Autodesk Inventor part; units mm, degrees
ref_plane "YZ Plane" through (0, 0, 0) normal (1, 0, 0) x (0, 1, 0)
ref_plane "XZ Plane" through (0, 0, 0) normal (0, 1, 0) x (-1, 0, 0)
ref_plane "XY Plane" through (0, 0, 0) normal (0, 0, 1) x (1, 0, 0)
sketch "Sketch1" plane through (0, 0, 0) normal (0, 1, 0) x (-1, 0, 0)
  circle A0 centre (5.2854, 6.2781) radius 7.75
  point P0 (0, 0)
  dimension "d0" = 15.5
extrude "Extrusion1" add sketch "Sketch1" along normal blind 101.6
sketch "Sketch2" plane through (-5.2854, 101.6, 6.2781) normal (0, 1, 0) x (1, 0, 0)
  circle A0 centre (0, 0) radius 7.75 construction
  circle A1 centre (0, 0) radius 7
  point P0 (5.2854, 6.2781)
  dimension "d3" = 14
  dimension "d4" = 0
extrude "Extrusion2" cut sketch "Sketch2" against normal blind 101.6
sketch "Sketch3" plane through (-5.2854, 0, 6.2781) normal (0, -1, 0) x (1, 0, 0)
  circle A0 centre (0, 0) radius 7 construction
  line L0 (10, 17.5) -> (-10, 17.5)
  line L1 (-10, 17.5) -> (-10, -17.5)
  line L2 (-10, -17.5) -> (10, -17.5)
  line L3 (10, -17.5) -> (10, 17.5)
  circle A1 centre (2.5, 12) radius 2
  circle A2 centre (2.5, -12) radius 2
  point P0 (5.2854, -6.2781)
  dimension "d7" = 35
  dimension "d8" = 20
  dimension "d11" = 17.5
  dimension "d12" = 10
  dimension "d14" = 4
  dimension "d15" = 4
  dimension "d16" = 24
  dimension "d17" = 5.5
  dimension "d18" = 7.5
  dimension "d19" = 7.5
extrude "Extrusion3" add sketch "Sketch3" along normal blind 3
fillet "Fillet1" radius 2 4 edges at (-5.2854, 0, 23.7781) (-15.2854, 0, 6.2781) (-5.2854, 0, -11.2219) (4.7146, 0, 6.2781)
fillet "Fillet2" radius 2 1 edges at (2.4646, 101.6, 6.2781)
properties part number "Flag Holder"
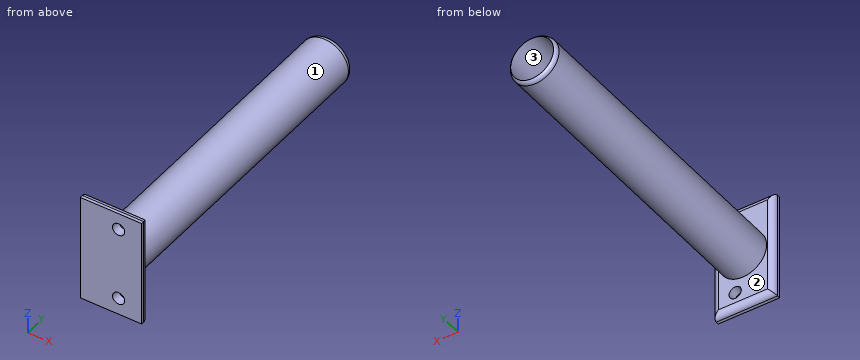
Source: CAD feature listing. Evaluate the final solid. Frame: model axes, mm. Face numbers are marked on the shaded views. Coordinates: 2 decimals unless noted, no trailing zeros. Order: outer loops, then holes, each group sorted by start corner. A loop starts at its lowest first (then second) coordinate and runs counter-clockwise, first axis right, second up.
Item 1: Cut plane B-B (y = 10.5). Return loops of the section in (x, z), plus the area to 3 significant figures.
Output values:
outline: circle Ø15.5 at (-5.29, 6.28); hole circle Ø14 at (-5.29, 6.28)
area: 34.8 mm2
Item 2: Material intervals for line 1 (X direction, y = 5.5, z = 6.5); line 2 (Z direction, x = -5, y = 11); line 3 (Y direction, x = -6.25, z = -4), sorted ascending.
Output values:
line 1: x = -13.03 to -12.28, 1.71 to 2.46
line 2: z = -1.47 to -0.72, 13.27 to 14.02
line 3: y = -3 to 0
Item 3: Cut plane A-A (x = -3.5). Count the separate pieces of the cut face and the enclosed holes in it, plus the area to 3 significant figures.
Output values:
separate pieces: 3
enclosed holes: 0
area: 237 mm2
Item 4: Pull-direction query (Z, two-part tool) for the marked faces 1, 2 and 3; classes: pulls with the +Z half, pulls with the -Z half, needs draft (parallel to the pull), parting line crosses it, or undercut.
Output values:
face 1: parting line crosses it
face 2: needs draft
face 3: undercut
Item 5: First-contact query: P1, Ø3, axis at y = 14, z = 4.5, coming from the +X side; P2, Ø4, axis at y = 76.5, z = 8.5, coming from the -X side; P3, Ø4.5, axis at x = -2.79, z = 18.28, coming from the -Y side; P4, Ø3, axis at y = 52.5, z = 9.5, coming from the -X side. Flat tips, straight axial feed; report the tip coordinate or a pass-through.
Output values:
P1: stops at x = 2.46
P2: stops at x = -13.03
P3: stops at y = -3
P4: stops at x = -12.84
